CAD build for the part. Positions are in the model's coordinates, mm. A direction names the side the tool comes from. Round coordinates to 2 decimals unless told otherwise and drop trailing zeros. Order: outer loops, then holes, each group sorted by start corner. A loop starts at its lowest first (then second) coordinate and runs counter-clockwise, first axis right, second up. Notation, with made-up numbers: (-2.5, 47) -> (44.5, 47) arc R21 cw to (44.5, 52) -> close; hole circle Ø11 at (53, 58). An arc over 180 degrees is marked (long way). Return JSON: item names as keys, results as strings. Group by question number.
Q1. Which spindle directions (+Z, -Z, +X, -X, +Y, -Y) get a long thin tool onto all of the face, cutting with end or side? Do faces 5 (the flat face through (939, 120, 65)), 6 (the flat face through (939, 21, 90)), 7 (the conical face through (-50.787, 21.057, 143.767)), 8 (the flat face through (939, -80, 65)). Say none if no direction does.
Q2. Flat gauge pins, fed straight in: pin 1 (6 mm diameter, centred on x = 806.5, y = -85, fed in from -Z); pin 2 (2 mm diameter, centred on x = 645, y = 91.5, fed in from +Z); pin 3 (15 mm diameter, centred on x = 918, z = 76, fed in from -Y); pin 4 (15 mm diameter, centred on x = 952.5, z = 56, fed in from +Y). Where does each tip first touch, or does it go through?
Q3. Mould opens along Z. For faces 1 (the flat face through (-41, -64, 100)), 2 (the cylindrical face through (-28, -45, 327)), 3 (the flat face through (939, 21, 40)), 4 (the conical face through (11.41, 51.39, 142.51)) say: +Z half, -Z half, draft (parallel to the pull), parting line (faces both ways), or undercut.
Q4. Cut at C-C (x = 0). Write the cut outline in (y, z), then the cut area to 3 significant figures.
Q5. Probe line 1 along X through (y, z) = (0, 414); line 2 along Y through (x, z) = (0, 304); line 3 along X through (y, z) = (32.5, 286.5). List the from-to ranges inside material, lowest first.
Q6. Cut at D-D (y = 0). Write the cut outline in (x, z), then the cut area to 3 significant figures.
Q7. Cut at A-A (z = 187.5). Write the cut outline in (x, y), then the cut area to 3 significant figures.
Q8. Cut at B-B (y = 98.5). Write the cut outline in (x, z), then the cut area to 3 significant figures.
from build123d import *

# Parameters (mm, degrees)
BOX001_W     = 100
BOX001_H     = 200
BOX001_DEPTH = 50
BOX_W        = 1000
BOX_H        = 300
BOX_DEPTH    = 500
SKETCH001_R  = 50
PAD_DEPTH    = 100


with BuildPart() as box001:
    # Box001 → Box001 (new body)
    with BuildSketch(Plane(origin=(890, -80, 40), x_dir=(1, 0, 0), z_dir=(0, 0, 1))):
        with Locations((50, 100)):
            Rectangle(BOX001_W, BOX001_H)
    extrude(amount=BOX001_DEPTH)


with BuildPart() as body:
    # Sketch → Revolution (revolve)
    with BuildSketch(Plane.XZ):
        with BuildLine():
            Line((-50, 649.259148), (-50, 150))
            ThreePointArc((-51.149586, 145.344876), (-50.29165, 147.602515), (-50, 150))
            Line((-51.149586, 145.344876), (-75, 100))
            Line((-75, 100), (-78, 100))
            Line((-78, 100), (-53.804711, 146.000561))
            ThreePointArc((-53.804711, 146.000561), (-53.204155, 147.580909), (-53, 149.259148))
            Line((-53, 149.259148), (-53, 649.259148))
            Line((-53, 649.259148), (-50, 649.259148))
        make_face()
    revolve(axis=Axis((0, 0, 0), (0, 0, 1)))


with BuildPart() as fusion:
    # Box → Box (new body)
    with BuildSketch(Plane(origin=(-110, -140, 0), x_dir=(1, 0, 0), z_dir=(0, 0, 1))):
        with Locations((500, 150)):
            Rectangle(BOX_W, BOX_H)
    extrude(amount=BOX_DEPTH)

    # Cut: cut Body
    add(body.part, mode=Mode.SUBTRACT)

    # Sketch001 (on Face14 of BaseFeature) → Pad (new body)
    with BuildSketch(Plane.XY.offset(500)):
        Circle(SKETCH001_R)
    extrude(amount=PAD_DEPTH)

    # Fusion: union Box001
    add(box001.part)


solid = fusion.part
Solution:
{
 "1": {"face 5": "+Z, -Z, +X, +Y", "face 6": "+Z, +X, +Y, -Y", "face 7": "none", "face 8": "+Z, -Z, +X, -Y"},
 "2": {"pin 1": "stops at z = 0", "pin 2": "stops at z = 500", "pin 3": "stops at y = -80", "pin 4": "stops at y = 120"},
 "3": {"face 1": "undercut", "face 2": "draft", "face 3": "-Z half", "face 4": "undercut"},
 "4": {"outline": "(-140, 0) -> (160, 0) -> (160, 500) -> (53, 500) -> (53, 149.26) arc R7 ccw to (53.8, 146) -> (78, 100) -> (75, 100) -> (51.15, 145.34) arc R10 cw to (50, 150) -> (50, 600) -> (-50, 600) -> (-50, 150) arc R10 cw to (-51.15, 145.34) -> (-75, 100) -> (-78, 100) -> (-53.8, 146) arc R7 ccw to (-53, 149.26) -> (-53, 500) -> (-140, 500) -> close", "area": "158,000 mm²"},
 "5": {"line 1": "x = -110 to -53, -50 to 50, 53 to 890", "line 2": "y = -140 to -53, -50 to 50, 53 to 160", "line 3": "x = -110 to -41.87, -38 to 38, 41.87 to 890"},
 "6": {"outline": "(-110, 0) -> (890, 0) -> (890, 40) -> (990, 40) -> (990, 90) -> (890, 90) -> (890, 500) -> (53, 500) -> (53, 149.26) arc R7 ccw to (53.8, 146) -> (78, 100) -> (75, 100) -> (51.15, 145.34) arc R10 cw to (50, 150) -> (50, 600) -> (-50, 600) -> (-50, 150) arc R10 cw to (-51.15, 145.34) -> (-75, 100) -> (-78, 100) -> (-53.8, 146) arc R7 ccw to (-53, 149.26) -> (-53, 500) -> (-110, 500) -> close", "area": "513,000 mm²"},
 "7": {"outline": "(-110, -140) -> (890, -140) -> (890, 160) -> (-110, 160) -> close; circle Ø100 at (0, 0); hole circle Ø106 at (0, 0)", "area": "299,000 mm²"},
 "8": {"outline": "(-110, 0) -> (890, 0) -> (890, 40) -> (990, 40) -> (990, 90) -> (890, 90) -> (890, 500) -> (-110, 500) -> close", "area": "505,000 mm²"}
}
